Can you work these out from the model? Positions are in its coordinate system, mm. Give positions to 0.01 mm unless a question says otherwise; leave off trailing zeros. Write each loop counter-clockwise with the first axis right and the second up, starting at its lowest first coordinate (ties: lowest second). Pieces come first, ordered by that corner, then holes. Notation, with made-up numbers: (-6, -22) - (5, -22) arc R24 cw to (5, -3) - close; hole circle Ø8 at (50, 38.5). An arc over 180 degrees is marked (long way). Use a Markdown table: item, result. Add a question column.
```python
from build123d import *

# Parameters (mm, degrees)
F0_W     = 2000
F0_H     = 1000
F0_W_2   = 1860
F0_H_2   = 860
F1_DEPTH = 25
F2_W     = 360
F2_H     = 30
F3_DEPTH = 25
F4_SCALE = 0.4


with BuildPart() as f1:
    # F0 (on Front) → F1 (new body)
    with BuildSketch(Plane.XZ):
        with Locations((1000, -500)):
            Rectangle(F0_W, F0_H)
        with Locations((1000, -500)):
            Rectangle(F0_W_2, F0_H_2, mode=Mode.SUBTRACT)
    extrude(amount=F1_DEPTH)

    # F2 (on face) → F3 (join)
    with BuildSketch(Plane.XZ.offset(25)):
        with Locations((380, -35)):
            Rectangle(F2_W, F2_H)
        with Locations((380, -965)):
            Rectangle(F2_W, F2_H)
    extrude(amount=F3_DEPTH)


with BuildPart() as f1_1:
    # F4: moved
    add(f1.part.scale(F4_SCALE).moved(Location((1200, -15, -600))))


solid = f1_1.part
```
Q1. If I drill on probe 1 along Z at (x, y) = (1318.5, -21); probe 2 along X at (y, z) = (-22.5, -724), over which ranges is the centre line in solid material (lowest first)? Write a range as [from, to].
Q2. Suppose I cut it at C-C (z = -739). Please give me the cut outline in (x, y), and give its area (3 significant figures).
Q3. Suppose I cut it at A-A (y = -28). Please give me the cut outline in (x, z), and give its area (3 significant figures).
Q4. Suppose I cut it at B-B (x = 1390). Please give me the cut outline in (y, z).
Q5. I'm going to push flat-ended pins straight in: P1, Ø8, axis at y = -32, z = -614.5, coming from the +X side; P2, Ø6, axis at x = 1320, y = -33, coming from the -Z side; P3, Ø3, axis at x = 1356.5, y = -32, coming from the +Z side. Where does each tip first touch, or does it pass through?
Derived:
| question | item | result |
|---|---|---|
| 1 | probe 1 | [-1000, -972], [-628, -600] |
| 1 | probe 2 | [1200, 1228], [1972, 2000] |
| 2 | outline | (1200, -25) - (1228, -25) - (1228, -15) - (1200, -15) - close; (1972, -25) - (2000, -25) - (2000, -15) - (1972, -15) - close |
| 2 | area | 560 mm² |
| 3 | outline | (1280, -992) - (1424, -992) - (1424, -980) - (1280, -980) - close; (1280, -620) - (1424, -620) - (1424, -608) - (1280, -608) - close |
| 3 | area | 3,460 mm² |
| 4 | outline | (-35, -992) - (-25, -992) - (-25, -1000) - (-15, -1000) - (-15, -972) - (-25, -972) - (-25, -980) - (-35, -980) - close; (-35, -620) - (-25, -620) - (-25, -628) - (-15, -628) - (-15, -600) - (-25, -600) - (-25, -608) - (-35, -608) - close |
| 5 | P1 | x = 1424 |
| 5 | P2 | z = -992 |
| 5 | P3 | z = -608 |
